Verification items for the finished model (mm, model axes). A direction names the side the tool comes from. Give positions to 0.01 mm unless a question says otherwise; leave off trailing zeros. Write each loop counter-clockwise with the first axis right and the second up, starting at its lowest first coordinate (ties: lowest second). Pieces come first, ordered by that corner, then holes. Notation, with made-up numbers: (-20.5, 30.5) -> (28.5, 30.5) arc R12 cw to (28.5, 53.5) -> close; hole circle Ø4 at (6.5, 15). An arc over 180 degrees is marked (long way). Answer as CSV lines item,"result". Start each with the question number.
1) Material ranges on L1, parallel to X at y = -21.5, z = 0.4; L2, parallel to X at y = -23, z = 2.9; L3, parallel to X at y = -25, z = 2.7, recorded low to high.
2) Gauge pin test, flat ends, axial feed: pin 1 Ø1.5 at (x, y) = (-23, -26) entering from -Z; pin 2 Ø4 at (x, y) = (15.95, -25) entering from +Z. Record the tip position at first contact, or that the pin passes through.
3) Sectioned sample at D-D on y = -6. Record the cut outline in (x, z).
4) Sectioned sample at A-A on y = -25. Give the number of separate pieces and of enclosed holes in the cut face, and give its area (3 significant figures).
5) Tool access check on faces 1 (the flat face through (10.55, -24, 1)), 2 (the flat face through (-18, -24, 0)). Record the directions out of +Z, -Z, +X, -X, +Y, -Y that give a thin tool (end or side, any length) a straight path to the whole face; none if there is none.
6) Sectioned sample at C-C on z = 0.9. Record the cut outline in (x, y).
```python
from build123d import *

# Parameters (mm, degrees)
F1_DEPTH      = 49
F2_R          = 1.5
F3_DEPTH      = 25
F3_DEPTH_BACK = 25
F4_DEPTH      = 12.4
F5_SIZE       = 3.99999


# Not quite as in the source:
# - a fillet or chamfer is up to 0.001 mm smaller than in the source, because OpenCascade refuses the exact size
# - a feature names something its author has since deleted; it is built from what else it names


with BuildPart() as f1:
    # F0 (on Front) → F1 (new body)
    with BuildSketch(Plane.XZ):
        Polygon((-16.275, 4), (-32.55, 4), (-32.55, 0), (-26.55, 0), (-26.55, 2.2), (-21.45, 2.2), (-21.45, 0), (-16.275, 0), align=None)
        Polygon((0, 4), (-16.275, 4), (-16.275, 0), (-10.55, 0), (-10.55, 2.2), (-5.45, 2.2), (-5.45, 0), (0, 0), align=None)
        Polygon((16.275, 4), (0, 4), (0, 0), (5.45, 0), (5.45, 2.2), (10.55, 2.2), (10.55, 0), (16.275, 0), align=None)
        Polygon((32.55, 4), (16.275, 4), (16.275, 0), (21.45, 0), (21.45, 2.2), (26.55, 2.2), (26.55, 0), (32.55, 0), align=None)
    extrude(amount=F1_DEPTH)

    # F2 (on Top) → F3 (cut, two sides)
    with BuildSketch(Plane.XY) as f3_sk:
        with Locations((-15.95, -25)):
            Circle(F2_R)
    extrude(amount=-F3_DEPTH, mode=Mode.SUBTRACT)
    extrude(f3_sk.sketch, amount=F3_DEPTH_BACK, mode=Mode.SUBTRACT)

    # F2 (on Top) → F4 (cut)
    with BuildSketch(Plane.XY):
        with Locations((-15.95, -25)):
            Circle(F2_R)
        with Locations((15.95, -25)):
            Circle(F2_R)
    extrude(amount=F4_DEPTH, mode=Mode.SUBTRACT)

    # F5 (size 4 in the source; OpenCascade refuses exactly that, so slightly less here)
    f5_edges = [f1.edges().sort_by_distance(p)[0] for p in [
        (14.45, -25, 4),
        (-17.45, -25, 4),
    ]]
    chamfer(f5_edges, length=F5_SIZE)


solid = f1.part
```
Ans:
1,L1,"x = -32.55 to -26.55, -21.45 to -10.55, -5.45 to 5.45, 10.55 to 21.45, 26.55 to 32.55"
1,L2,"x = -32.55 to -19.87, -12.03 to 12.03, 19.87 to 32.55"
1,L3,"x = -32.55 to -20.15, -11.75 to 11.75, 20.15 to 32.55"
2,pin 1,"stops at z = 2.2"
2,pin 2,"stops at z = 0.5"
3,outline,"(-32.55, 0) -> (-26.55, 0) -> (-26.55, 2.2) -> (-21.45, 2.2) -> (-21.45, 0) -> (-10.55, 0) -> (-10.55, 2.2) -> (-5.45, 2.2) -> (-5.45, 0) -> (5.45, 0) -> (5.45, 2.2) -> (10.55, 2.2) -> (10.55, 0) -> (21.45, 0) -> (21.45, 2.2) -> (26.55, 2.2) -> (26.55, 0) -> (32.55, 0) -> (32.55, 4) -> (-32.55, 4) -> close"
4,separate pieces,"3"
4,enclosed holes,"0"
4,area,"160 mm²"
5,face 1,"-Z, +Y, -Y"
5,face 2,"-Z, +X, -X, +Y, -Y"
6,outline,"(-32.55, -49) -> (-26.55, -49) -> (-26.55, 0) -> (-32.55, 0) -> close; (-21.45, -49) -> (-10.55, -49) -> (-10.55, 0) -> (-21.45, 0) -> close; (-5.45, -49) -> (5.45, -49) -> (5.45, 0) -> (-5.45, 0) -> close; (10.55, -49) -> (21.45, -49) -> (21.45, 0) -> (10.55, 0) -> close; (26.55, -49) -> (32.55, -49) -> (32.55, 0) -> (26.55, 0) -> close; hole circle Ø4.8 at (-15.95, -25); hole circle Ø4.8 at (15.95, -25)"
